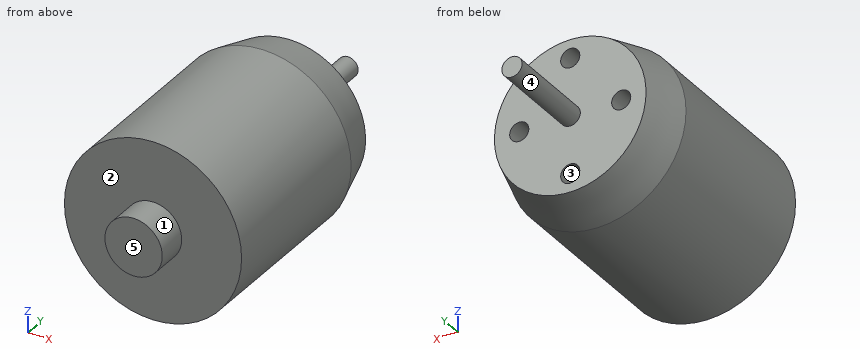
```python
from build123d import *

# Parameters (mm, degrees)
SKETCH1_R           = 13.9
BOSS_EXTRUDE1_DEPTH = 35.2
SKETCH2_R           = 1.585
BOSS_EXTRUDE2_DEPTH = 15
SKETCH4_R           = 1.5
CUT_EXTRUDE1_DEPTH  = 7
CHAMFER1_SIZE       = 7
CHAMFER1_SIZE2      = 2
SKETCH5_R           = 4.5
BOSS_EXTRUDE3_DEPTH = 5


with BuildPart() as part:
    # Sketch1 → Boss-Extrude1 (new body)
    with BuildSketch(Plane(origin=(0, 0, 0), x_dir=(1, 0, 0), z_dir=(0, 1, 0))):
        with Locations(Location((0, 0, 0), (0, 0, 270))):
            Circle(SKETCH1_R)
    extrude(amount=BOSS_EXTRUDE1_DEPTH)

    # Sketch2 → Boss-Extrude2 (add)
    with BuildSketch(Plane(origin=(0, 35.2, 0), x_dir=(1, 0, 0), z_dir=(0, 1, 0))):
        with Locations(Location((0, 0, 0), (0, 0, 270))):
            Circle(SKETCH2_R)
    extrude(amount=BOSS_EXTRUDE2_DEPTH)

    # Sketch4 → Cut-Extrude1 (cut)
    with BuildSketch(Plane(origin=(0, 35.2, 0), x_dir=(1, 0, 0), z_dir=(0, 1, 0))):
        with Locations(Location((0, 9, 0), (0, 0, 270))):
            Circle(SKETCH4_R)
        with Locations(Location((-8, 0, 0), (0, 0, 270))):
            Circle(SKETCH4_R)
        with Locations(Location((8, 0, 0), (0, 0, 270))):
            Circle(SKETCH4_R)
        with Locations(Location((0, -9, 0), (0, 0, 270))):
            Circle(SKETCH4_R)
    extrude(amount=-CUT_EXTRUDE1_DEPTH, mode=Mode.SUBTRACT)

    # Chamfer1
    chamfer1_edges = [part.edges().sort_by_distance(p)[0] for p in [
        (0, 35.2, -13.9),
    ]]
    chamfer1_side = [part.faces().sort_by_distance(p)[0] for p in [
        (0, 17.6, -13.9),
    ]]
    chamfer(chamfer1_edges, length=CHAMFER1_SIZE, length2=CHAMFER1_SIZE2, reference=chamfer1_side[0])

    # Sketch5 → Boss-Extrude3 (add)
    with BuildSketch(Plane.XZ):
        with Locations(Location((0, 0, 0), (0, 0, 270))):
            Circle(SKETCH5_R)
    extrude(amount=BOSS_EXTRUDE3_DEPTH)


solid = part.part
```
Here's how the part is built. I have some questions about the finished solid (model axes, mm). Face numbers are marked on the shaded views. A direction names the side the tool comes from. Coordinates: 2 decimals unless noted, no trailing zeros. Write each loop counter-clockwise with the first axis right and the second up, starting at its lowest first coordinate (ties: lowest second). Pieces come first, ordered by that corner, then holes. Notation, with made-up numbers: (87, 12) -> (107, 12) arc R30 ccw to (107, 36) -> close; hole circle Ø3 at (19.25, 72). An arc over 180 degrees is marked (long way). Use a Markdown table: item, result. Add a question column.
(1) Please list where these lines run through material, in increasing order: line 1 (X direction, y = 31, z = 0); line 2 (Y direction, x = -7.25, z = -6.5); line 3 (Y direction, x = -7.25, z = -0.75).
(2) We'd pull the mould along Z, two halves only. Please class the marked faces 1, 2 and 3: +Z half, -Z half, draft (parallel to the pull), parting line (faces both ways), or undercut.
(3) If we section it at A-A, the plane z = 0: Write out the boundary of the cut face in (x, y) (3 decimals), and give its area (3 significant figures).
(4) If we section it at C-C, the plane y = 27.5: Write out the boundary of the cut face in (x, z), and give its area (3 significant figures).
(5) For the marked faces 4 and 5, which set-ups out of +Z, -Z, +X, -X, +Y, -Y let a thin tool reach every point of the face, with its end or its side?
(6) If we section it at B-B, the plane y = 34: Write out the boundary of the cut face in (x, z), and give its area (3 significant figures).
(7) I'm going to push flat-ended pins straight in: P1, Ø2.5, axis at x = 0.5, z = -9, coming from the +Y side; P2, Ø1, axis at y = 5.5, z = 10.5, coming from the -X side; P3, Ø5, axis at x = 7.5, z = 4.5, coming from the -Y side. Where does each tip first touch, or does it pass through?
Outcome:
| question | item | result |
|---|---|---|
| 1 | line 1 | x = -13.1 to -9.5, -6.5 to 6.5, 9.5 to 13.1 |
| 1 | line 2 | y = 0 to 35.2 |
| 1 | line 3 | y = 0 to 28.2 |
| 2 | face 1 | parting line |
| 2 | face 2 | draft |
| 2 | face 3 | undercut |
| 3 | outline | (-13.9, 0) -> (-4.5, 0) -> (-4.5, -5) -> (4.5, -5) -> (4.5, 0) -> (13.9, 0) -> (13.9, 28.2) -> (11.9, 35.2) -> (9.5, 35.2) -> (9.5, 28.2) -> (6.5, 28.2) -> (6.5, 35.2) -> (1.585, 35.2) -> (1.585, 50.2) -> (-1.585, 50.2) -> (-1.585, 35.2) -> (-6.5, 35.2) -> (-6.5, 28.2) -> (-9.5, 28.2) -> (-9.5, 35.2) -> (-11.9, 35.2) -> (-13.9, 28.2) -> close |
| 3 | area | 1,020 mm^2 |
| 4 | outline | circle Ø27.8 at (0, 0) |
| 4 | area | 607 mm^2 |
| 5 | face 4 | +Y |
| 5 | face 5 | +Z, -Z, +X, -X, -Y |
| 6 | outline | circle Ø24.49 at (0, 0); hole circle Ø3 at (-8, 0); hole circle Ø3 at (0, -9); hole circle Ø3 at (0, 9); hole circle Ø3 at (8, 0) |
| 6 | area | 443 mm^2 |
| 7 | P1 | stops at y = 35.2 |
| 7 | P2 | stops at x = -9.65 |
| 7 | P3 | stops at y = 0 |
